Source: CAD feature listing. Evaluate the final solid. Frame: model axes, mm. Give positions to 0.01 mm unless a question says otherwise; leave off trailing zeros. Order: outer loops, then holes, each group sorted by start corner. A loop starts at its lowest first (then second) coordinate and runs counter-clockwise, first axis right, second up.
```python
from build123d import *

# Parameters (mm, degrees)
F0_W        = 300
F0_H        = 180
F0_R        = 10
F1_DEPTH    = 25
F2_SIZE2    = 2
F2_SIZE     = 2
F3_SIZE2    = 2
F3_SIZE     = 2
F4_T1_DEPTH = 71


# Not quite as in the source:
# - a fillet or chamfer that OpenCascade refuses, or shapes differently, is made with other operations: its cross-section is extruded or revolved along the edge and cut away or added


with BuildPart() as f1:
    # F0 (on Top) → F1 (new body)
    with BuildSketch(Plane.XY):
        Rectangle(F0_W, F0_H)
        with Locations((-125, -65)):
            Circle(F0_R, mode=Mode.SUBTRACT)
        with Locations((0, -65)):
            Circle(F0_R, mode=Mode.SUBTRACT)
        with Locations((125, -65)):
            Circle(F0_R, mode=Mode.SUBTRACT)
        with Locations((-125, 65)):
            Circle(F0_R, mode=Mode.SUBTRACT)
        with Locations((0, 65)):
            Circle(F0_R, mode=Mode.SUBTRACT)
        with Locations((125, 65)):
            Circle(F0_R, mode=Mode.SUBTRACT)
    extrude(amount=F1_DEPTH)

    # F2
    f2_edges = [f1.edges().sort_by_distance(p)[0] for p in [
        (-135, -65, 25),
        (-135, 65, 25),
        (-10, -65, 25),
        (-10, 65, 25),
        (115, 65, 25),
        (115, -65, 25),
        (-150, 0, 25),
        (-150, 0, 0),
        (150, 0, 25),
        (150, 0, 0),
    ]]
    chamfer(f2_edges, length=F2_SIZE, length2=F2_SIZE2)

    # F3
    f3_edges = [f1.edges().sort_by_distance(p)[0] for p in [
        (0, -90, 25),
        (0, -90, 0),
        (0, 90, 25),
        (0, 90, 0),
    ]]
    chamfer(f3_edges, length=F3_SIZE, length2=F3_SIZE2)

    # F4: fillet of radius 10 on 4 edges, made by hand

    # F4_s2 → F4_t1 (cut)
    with BuildSketch(Plane.XY.offset(-23)):
        with BuildLine():
            ThreePointArc((150, -80), (147.0710678119, -87.0710678119), (140, -90))
            Line((140, -90), (150, -90))
            Line((150, -90), (150, -80))
        make_face()
        with BuildLine():
            ThreePointArc((-150, -80), (-147.0710678119, -87.0710678119), (-140, -90))
            Line((-140, -90), (-150, -90))
            Line((-150, -90), (-150, -80))
        make_face()
        with BuildLine():
            ThreePointArc((-140, 90), (-147.0710678119, 87.0710678119), (-150, 80))
            Line((-150, 80), (-150, 90))
            Line((-150, 90), (-140, 90))
        make_face()
        with BuildLine():
            ThreePointArc((140, 90), (147.0710678119, 87.0710678119), (150, 80))
            Line((150, 80), (150, 90))
            Line((150, 90), (140, 90))
        make_face()
    extrude(amount=F4_T1_DEPTH, mode=Mode.SUBTRACT)


solid = f1.part
```
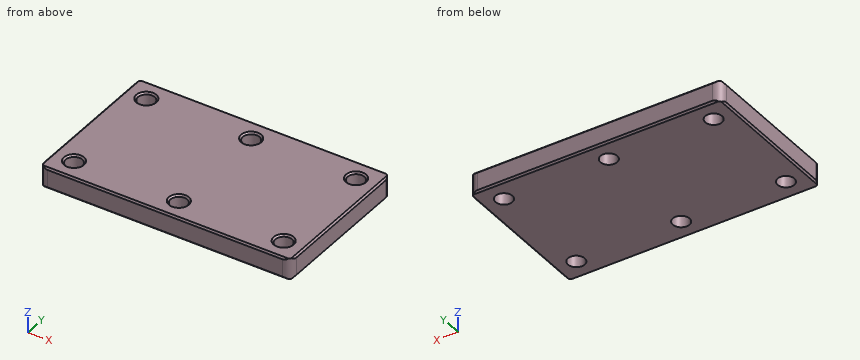
1) Section query C-C, the plane z = 14.75. Return the cut outline in (x, y), and give its area (3 significant figures).
Report:
outline: (-150, -80) arc R10 ccw to (-140, -90) - (140, -90) arc R10 ccw to (150, -80) - (150, 80) arc R10 ccw to (140, 90) - (-140, 90) arc R10 ccw to (-150, 80) - close; hole circle Ø20 at (-125, -65); hole circle Ø20 at (-125, 65); hole circle Ø20 at (0, -65); hole circle Ø20 at (0, 65); hole circle Ø20 at (125, -65); hole circle Ø20 at (125, 65)
area: 52,000 mm2
2) Section query A-A, the plane x = -125. Return the cut outline in (y, z).
Report:
outline: (-90, 2) - (-88, 0) - (-75, 0) - (-75, 23) - (-77, 25) - (-88, 25) - (-90, 23) - close; (-55, 0) - (55, 0) - (55, 23) - (53, 25) - (-53, 25) - (-55, 23) - close; (75, 0) - (88, 0) - (90, 2) - (90, 23) - (88, 25) - (77, 25) - (75, 23) - close
3) Section query B-B, the plane y = 65. Return the cut outline in (x, z), and give its area (3 significant figures).
Report:
outline: (-150, 2) - (-148, 0) - (-135, 0) - (-135, 23) - (-137, 25) - (-148, 25) - (-150, 23) - close; (-115, 0) - (-10, 0) - (-10, 23) - (-12, 25) - (-113, 25) - (-115, 23) - close; (10, 0) - (115, 0) - (115, 23) - (113, 25) - (12, 25) - (10, 23) - close; (135, 0) - (148, 0) - (150, 2) - (150, 23) - (148, 25) - (137, 25) - (135, 23) - close
area: 5,980 mm2
4) Section query D-D, the plane x = 125.5. Count the separate pieces of the cut face and the enclosed holes in it, and give its area (3 significant figures).
Report:
separate pieces: 3
enclosed holes: 0
area: 3,490 mm2
5) Material intervals for L1, parallel to Y at x = 0, z = 17.5, sorted ascending.
Report:
L1: y = -90 to -75, -55 to 55, 75 to 90
